The model under review builds one solid part; all positions refer to its coordinate system, in mm. Face numbers are marked on the shaded views. A direction names the side the tool comes from. Give positions to 0.01 mm unless a question says otherwise; leave off trailing zeros. Loops run counter-clockwise (first coordinate to the right, second up) from the corner with the lowest first, then second, coordinate; pieces in that order, holes last. Notation, with made-up numbers: M -2,55.5 L 47,55.5 A17 cw 47,60.5 Z; hole C -18.5,-19.75 d7. An arc over 180 degrees is marked long. Write item = value, one per line. Start each with the question number.
1. We need section A-A on x = 0. Give the boundary of the cut face in (y, z), then the cut area to 3 significant figures.
2. For the marked faces 4 and 5, list the 3-axis set-ups (+Z, -Z, +X, -X, +Y, -Y) from which the entire face can be reached by the end or side of a thin tool; tool diameter is ignored.
3. We need section C-C on z = 26. Give the boundary of the cut face in (x, y).
4. Wall thickness on line 1 along Z through (x, y) = (-21, -9.5); line 2 along Y through (x, z) = (8, 39); line 3 along Z through (x, y) = (-12.5, 27.5): over which ranges is each line inside the solid? List them lowest first. Write a range as from..to.
5. Draft analysis for pull direction X (two halves, no side actions). For the marked faces 1, 2 and 3, state which applies: pulls with the +X half, pulls with the -X half, needs draft (parallel to the pull), parting line crosses it, or undercut.
6. For pin 1 (2 mm diameter, centred on x = 12, z = 26.5, fed in from +Y); pin 2 (12 mm diameter, centred on x = -18, y = 33, fed in from +Z); pin 3 (7 mm diameter, centred on x = 19.4, z = 26.8, fed in from -Y), all flat-tipped, find the tip position at first contact; note any pin that passes through.
7. We need section D-D on x = -6.5. Give the boundary of the cut face in (y, z).
8. We need section B-B on y = 36.48. Give the boundary of the cut face in (x, z).
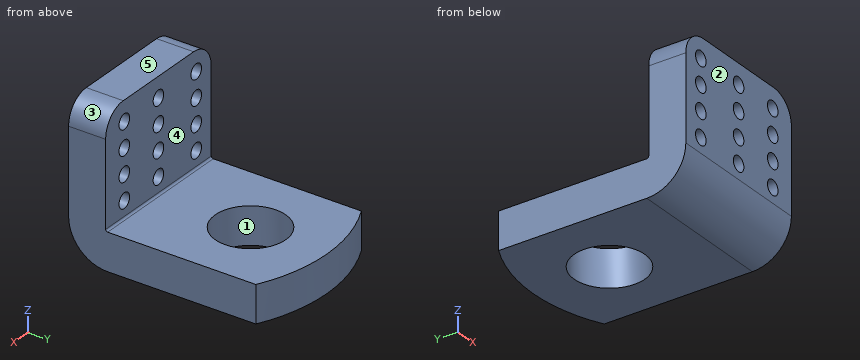
from build123d import *

# Parameters (mm, degrees)
SKETCH1_R          = 14.3
BASE_FLANGE1_DEPTH = 15
EDGE_FLANGE1_DEPTH = 60
SKETCH9_R          = 3
CUT_EXTRUDE1_DEPTH = 50
FILLET1_R          = 10


# Sheet-metal steps are written as plain solids
with BuildPart() as part:
    # Sketch1 → Base-Flange1 (new body)
    with BuildSketch(Plane.XY):
        with BuildLine():
            Line((-30, 0), (30, 0))
            Line((30, 0), (30, 60))
            ThreePointArc((30, 60), (0, 67.337187027), (-30, 60))
            Line((-30, 60), (-30, 0))
        make_face()
        with Locations((0, 36.48)):
            Circle(SKETCH1_R, mode=Mode.SUBTRACT)
    extrude(amount=-BASE_FLANGE1_DEPTH)

    # Edge-Flange1 section (across the edge) → Edge-Flange1 (add)
    with BuildSketch(Plane(origin=(-30, -0.8, 0), x_dir=(0, 1, 0), z_dir=(1, 0, 0))):
        with BuildLine():
            Line((-15, 0.8), (-15, 45))
            Line((-15, 45), (0, 45))
            Line((0, 45), (0, 0.8))
            ThreePointArc((0, 0.8), (0.234314575, 0.234314575), (0.8, 0))
            Line((0.8, 0), (0.8, -15))
            ThreePointArc((0.8, -15), (-10.372287143, -10.372287143), (-15, 0.8))
        make_face()
    extrude(amount=EDGE_FLANGE1_DEPTH)

    # Sketch9 → Cut-Extrude1 (cut)
    with BuildSketch(Plane(origin=(0, -0.8, 0), x_dir=(1, 0, 0), z_dir=(0, 1, 0))):
        with Locations(Location((-21.478093951, -6.800727635, 0), (0, 0, 270))):
            Circle(SKETCH9_R)
        with Locations(Location((19.398278521, -6.800727635, 0), (0, 0, 270))):
            Circle(SKETCH9_R)
        with Locations(Location((0, -6.800727635, 0), (0, 0, 270))):
            Circle(SKETCH9_R)
        with Locations(Location((-21.478093951, -16.800727635, 0), (0, 0, 270))):
            Circle(SKETCH9_R)
        with Locations(Location((-21.478093951, -26.800727635, 0), (0, 0, 270))):
            Circle(SKETCH9_R)
        with Locations(Location((-21.478093951, -36.800727635, 0), (0, 0, 270))):
            Circle(SKETCH9_R)
        with Locations(Location((0, -16.800727635, 0), (0, 0, 270))):
            Circle(SKETCH9_R)
        with Locations(Location((0, -26.800727635, 0), (0, 0, 270))):
            Circle(SKETCH9_R)
        with Locations(Location((0, -36.800727635, 0), (0, 0, 270))):
            Circle(SKETCH9_R)
        with Locations(Location((19.398278521, -16.800727635, 0), (0, 0, 270))):
            Circle(SKETCH9_R)
        with Locations(Location((19.398278521, -26.800727635, 0), (0, 0, 270))):
            Circle(SKETCH9_R)
        with Locations(Location((19.398278521, -36.800727635, 0), (0, 0, 270))):
            Circle(SKETCH9_R)
    extrude(amount=-CUT_EXTRUDE1_DEPTH, mode=Mode.SUBTRACT)

    # Fillet1
    fillet1_edges = [part.edges().sort_by_distance(p)[0] for p in [
        (-30, -8.3, 45),
        (30, -8.3, 45),
    ]]
    fillet(fillet1_edges, radius=FILLET1_R)


solid = part.part
Final values:
q1.outline = M -15.8,0.8 A15.8 ccw 0,-15 L 22.18,-15 L 22.18,0 L 0,0 A0.8 cw -0.8,0.8 L -0.8,3.8 L -15.8,3.8 Z; M -15.8,9.8 L -0.8,9.8 L -0.8,13.8 L -15.8,13.8 Z; M -15.8,19.8 L -0.8,19.8 L -0.8,23.8 L -15.8,23.8 Z; M -15.8,29.8 L -0.8,29.8 L -0.8,33.8 L -15.8,33.8 Z; M -15.8,39.8 L -0.8,39.8 L -0.8,45 L -15.8,45 Z; M 50.78,-15 L 67.34,-15 L 67.34,0 L 50.78,0 Z
q1.area = 1,080 mm²
q2.face_4 = +Z, +X, -X, +Y
q2.face_5 = +Z, +X, -X, +Y, -Y
q3.outline = M -30,-15.8 L -24.37,-15.8 L -24.37,-0.8 L -30,-0.8 Z; M -18.59,-15.8 L -2.89,-15.8 L -2.89,-0.8 L -18.59,-0.8 Z; M 2.89,-15.8 L 16.51,-15.8 L 16.51,-0.8 L 2.89,-0.8 Z; M 22.29,-15.8 L 30,-15.8 L 30,-0.8 L 22.29,-0.8 Z
q4.line_1 = -11.82..3.84, 9.76..13.84, 19.76..23.84, 29.76..33.84, 39.76..44.95
q4.line_2 = -15.8..-0.8
q4.line_3 = -15..0
q5.face_1 = undercut
q5.face_2 = needs draft
q5.face_3 = pulls with the +X half
q6.pin_1 = -0.8
q6.pin_2 = 0
q6.pin_3 = -15.8
q7.outline = M -15.8,0.8 A15.8 ccw 0,-15 L 23.74,-15 L 23.74,0 L 0,0 A0.8 cw -0.8,0.8 L -0.8,45 L -15.8,45 Z; M 49.22,-15 L 67.01,-15 L 67.01,0 L 49.22,0 Z
q8.outline = M -30,-15 L -14.3,-15 L -14.3,0 L -30,0 Z; M 14.3,-15 L 30,-15 L 30,0 L 14.3,0 Z
